Part model, mm, in its own coordinate system. A direction names the side the tool comes from. Give positions to 0.01 mm unless a question says otherwise; leave off trailing zeros. Order: outer loops, then holes, each group sorted by start corner. A loop starts at its lowest first (then second) coordinate and runs counter-clockwise, first axis right, second up.
from build123d import *

# Parameters (mm, degrees)
BOSS_EXTRUDE2_DEPTH = 25
BOSS_EXTRUDE3_START = 25
SKETCH1_3_R         = 2.5
BOSS_EXTRUDE3_DEPTH = 20
CUT_EXTRUDE1_DEPTH  = 130


with BuildPart() as part:
    # Sketch1 → Boss-Extrude2 (new body)
    with BuildSketch(Plane(origin=(0, 0, 0), x_dir=(1, 0, 0), z_dir=(0, 1, 0))):
        with BuildLine():
            Line((-45, 70), (45, 70))
            ThreePointArc((45, 70), (48.535533906, 68.535533906), (50, 65))
            Line((50, 65), (50, -65))
            ThreePointArc((50, -65), (48.535533906, -68.535533906), (45, -70))
            Line((45, -70), (-45, -70))
            ThreePointArc((-45, -70), (-48.535533906, -68.535533906), (-50, -65))
            Line((-50, -65), (-50, 65))
            ThreePointArc((-50, 65), (-48.535533906, 68.535533906), (-45, 70))
        make_face()
    extrude(amount=BOSS_EXTRUDE2_DEPTH)

    # Sketch1<3> → Boss-Extrude3 (add)
    with BuildSketch(Plane(origin=(0, 0, 0), x_dir=(1, 0, 0), z_dir=(0, 1, 0)).offset(BOSS_EXTRUDE3_START)):
        with BuildLine():
            Line((-45, 70), (45, 70))
            ThreePointArc((45, 70), (48.535533906, 68.535533906), (50, 65))
            Line((50, 65), (50, -65))
            ThreePointArc((50, -65), (48.535533906, -68.535533906), (45, -70))
            Line((45, -70), (-45, -70))
            ThreePointArc((-45, -70), (-48.535533906, -68.535533906), (-50, -65))
            Line((-50, -65), (-50, 65))
            ThreePointArc((-50, 65), (-48.535533906, 68.535533906), (-45, 70))
        make_face()
        with Locations(Location((-45, 65, 0), (0, 0, 270))):
            Circle(SKETCH1_3_R, mode=Mode.SUBTRACT)
        with Locations(Location((45, 65, 0), (0, 0, 270))):
            Circle(SKETCH1_3_R, mode=Mode.SUBTRACT)
        with Locations(Location((45, -65, 0), (0, 0, 270))):
            Circle(SKETCH1_3_R, mode=Mode.SUBTRACT)
        with Locations(Location((-45, -65, 0), (0, 0, 270))):
            Circle(SKETCH1_3_R, mode=Mode.SUBTRACT)
        with BuildLine():
            Line((-40.417424305, 67), (40.417424305, 67))
            ThreePointArc((40.417424305, 67), (41.464466094, 61.464466094), (47, 60.417424305))
            Line((47, 60.417424305), (47, -60.417424305))
            ThreePointArc((47, -60.417424305), (41.464466094, -61.464466094), (40.417424305, -67))
            Line((40.417424305, -67), (-40.417424305, -67))
            ThreePointArc((-40.417424305, -67), (-41.464466094, -61.464466094), (-47, -60.417424305))
            Line((-47, -60.417424305), (-47, 60.417424305))
            ThreePointArc((-47, 60.417424305), (-41.464466094, 61.464466094), (-40.417424305, 67))
        make_face(mode=Mode.SUBTRACT)
    extrude(amount=BOSS_EXTRUDE3_DEPTH)

    # Sketch2 → Cut-Extrude1 (cut)
    with BuildSketch(Plane.XY.offset(70)):
        with BuildLine():
            Line((-33.600286554, 5.152304199), (33.600286554, 5.152304199))
            add(Edge.make_bspline(
                [(33.600286554, 20.375134216), (37.254581283, 19.906525536), (39.744987875, 13.002442779), (37.255381919, 5.419067927), (33.600286554, 5.152304199)],
                knots=[0, 0, 0, 0, 0.5, 1, 1, 1, 1], degree=3))
            Line((33.600286554, 20.375134216), (-33.600286554, 20.375134216))
            add(Edge.make_bspline(
                [(-33.600286554, 20.375134216), (-37.254581283, 19.906525536), (-39.744987875, 12.865320549), (-37.255381919, 5.419067927), (-33.600286554, 5.152304199)],
                knots=[0, 0, 0, 0, 0.5, 1, 1, 1, 1], degree=3))
        make_face()
    extrude(amount=-CUT_EXTRUDE1_DEPTH, mode=Mode.SUBTRACT)


solid = part.part
Item 1: Drop flat-ended pins along their axis: P1, Ø2.5, axis at x = 45, z = 65.5, coming from the +Y side; P2, Ø4.5, axis at x = 45, z = 65, coming from the -Y side. Give the stop position or say it passes through.
Item 2: Which spindle directions (+Z, -Z, +X, -X, +Y, -Y) get a long thin tool onto all of the face, cutting with end or side? Do faces 4 (the face through (-1, 22, -70)), 5 (the face through (-1, 13, -60)), 6 (the face through (47, 35, -1)). Say none if no direction does.
Item 3: Band-saw the part on A-A on y = 33.5. List the corners of the cut face in (x, z), plus the area to 3 significant figures.
Item 4: Drill centre lines: probe 1 along X at (y, z) = (34, 65); probe 2 along Y at (x, z) = (9, -24); probe 3 along Z at (x, y) = (-8.5, 36). Where is each one in solid material? Low to high.
Item 5: Pull direction Z, two halves, no side cores. Call faces 1 (the face through (45, 25, 65)), 2 (the face through (48, 45, 5)), 3 (the face through (49, 22, 68)): released by +Z, released by -Z, zero draft, split by the parting line, or undercut.
Item 6: Band-saw the part on B-B on x = 9.5. List the corners of the cut face in (y, z), plus the area to 3 significant figures.
Working result:
1. P1: stops at y = 25
1. P2: stops at y = 0
2. face 4: -Z, +X, -X, +Y, -Y
2. face 5: +Z
2. face 6: +Y
3. outline: (-50, -65) arc R5 ccw to (-45, -70) - (45, -70) arc R5 ccw to (50, -65) - (50, 65) arc R5 ccw to (45, 70) - (-45, 70) arc R5 ccw to (-50, 65) - close; hole circle Ø5 at (-45, -65); hole circle Ø5 at (-45, 65); hole (-47, -60.42) arc R5 cw to (-40.42, -67) - (40.42, -67) arc R5 cw to (47, -60.42) - (47, 60.42) arc R5 cw to (40.42, 67) - (-40.42, 67) arc R5 cw to (-47, 60.42) - close; hole circle Ø5 at (45, -65); hole circle Ø5 at (45, 65)
3. area: 1,480 mm2
4. probe 1: x = -50 to -47.5, -42.5 to -40, 40 to 42.5, 47.5 to 50
4. probe 2: y = 0 to 5.15, 20.38 to 25
4. probe 3: z = -70 to -67, 67 to 70
5. face 1: undercut
5. face 2: zero draft
5. face 3: released by +Z
6. outline: (0, -70) - (45, -70) - (45, -67) - (25, -67) - (25, 67) - (45, 67) - (45, 70) - (20.38, 70) - (20.38, -60) - (5.15, -60) - (5.15, 70) - (0, 70) - close
6. area: 1,640 mm2
